Source: three-view drawing plus pictorial views. Frame: mm from the lowest corner of the part. A direction names the side the tool comes from. Round coordinates to 2 decimals unless told otherwise and drop trailing zeros. Write each loop counter-clockwise with the first axis right and the second up, starting at its lowest first coordinate (ties: lowest second). Pieces come first, ordered by that corner, then holes. Notation, with made-up numbers: M 2.25,10.25 L 49.25,10.25 A23 cw 49.25,37.25 Z; hole C 68.25,33 d5. An arc over 180 degrees is marked long. Answer as CSV lines item,"result". Start each with the question number.
Q1. Section query B-B on z = 8. Output: boundary loops of the cut face in (x, y).
Q2. Ray query, probe 1 along X at (y, z) = (3, 8); probe 2 along Z at (x, y) = (10.3, 1.3); probe 3 along Z at (x, y) = (10, 3). Return the intervals inside material, ascending.
Q3. First-contact query: pin 1 (3 mm diameter, centred on x = 4, y = 24.9, fed in from +Z); pin 2 (2 mm diameter, centred on x = 3, y = 24, fed in from -Z); pin 3 (5 mm diameter, centred on x = 46.5, z = 27.5, fed in from +Y); pin 4 (10.5 mm diameter, centred on x = 46.3, z = 8, fed in from +Y). Flat tips, straight axial feed; report the tip coordinate or a pass-through.
Q4. Section query A-A on x = 10.3. Output: boundary loops of the cut face in (y, z), and give its area (3 significant figures).
Q5. Reachability of the marked faces 1 and 2 from +Z, -Z, +X, -X, +Y, -Y: full face, straight path, thin tool, end or side. Return the list, or none.
Q6. Section query C-C on y = 15. Output: boundary loops of the cut face in (x, z), and give its area (3 significant figures).
Q7. Section query D-D on y = 20. Output: boundary loops of the cut face in (x, z), and give its area (3 significant figures).
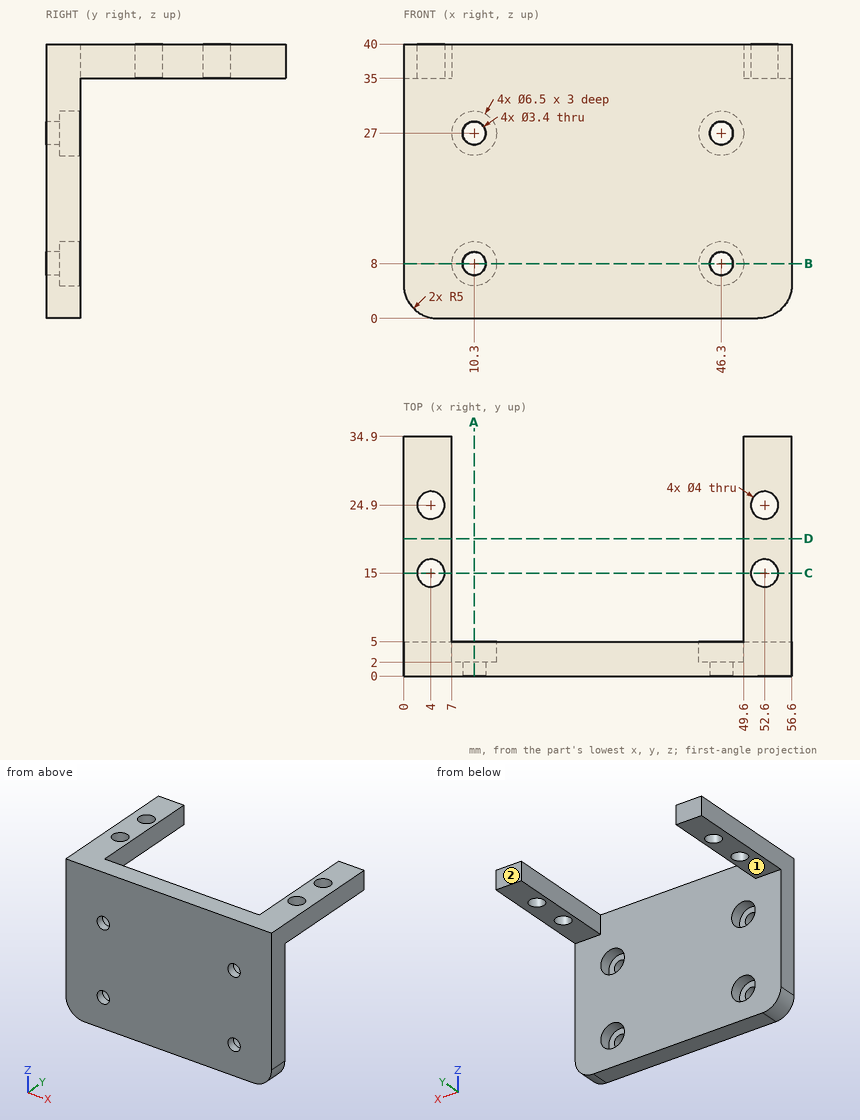
Entries:
1,outline,"M 0,0 L 8.6,0 L 8.6,2 L 7.05,2 L 7.05,5 L 0,5 Z; M 12,0 L 44.6,0 L 44.6,2 L 43.05,2 L 43.05,5 L 13.55,5 L 13.55,2 L 12,2 Z; M 48,0 L 56.6,0 L 56.6,5 L 49.55,5 L 49.55,2 L 48,2 Z"
2,probe 1,"x = 0 to 7.05, 13.55 to 43.05, 49.55 to 56.6"
2,probe 2,"z = 0 to 6.3, 9.7 to 25.3, 28.7 to 40"
2,probe 3,"z = 0 to 4.76, 11.24 to 23.76, 30.24 to 40"
3,pin 1,"passes through"
3,pin 2,"stops at z = 35"
3,pin 3,"stops at y = 2"
3,pin 4,"stops at y = 5"
4,outline,"M 0,0 L 5,0 L 5,4.75 L 2,4.75 L 2,6.3 L 0,6.3 Z; M 0,9.7 L 2,9.7 L 2,11.25 L 5,11.25 L 5,23.75 L 2,23.75 L 2,25.3 L 0,25.3 Z; M 0,28.7 L 2,28.7 L 2,30.25 L 5,30.25 L 5,40 L 0,40 Z"
4,area,"147 mm^2"
5,face 1,"-Z, +X, -X, +Y"
5,face 2,"+Z, -Z, +X, -X, +Y"
6,outline,"M 0,35 L 2,35 L 2,40 L 0,40 Z; M 6,35 L 7,35 L 7,40 L 6,40 Z; M 49.6,35 L 50.6,35 L 50.6,40 L 49.6,40 Z; M 54.6,35 L 56.6,35 L 56.6,40 L 54.6,40 Z"
6,area,"30.0 mm^2"
7,outline,"M 0,35 L 7,35 L 7,40 L 0,40 Z; M 49.6,35 L 56.6,35 L 56.6,40 L 49.6,40 Z"
7,area,"70.0 mm^2"
